```python
from build123d import *

# Parameters (mm, degrees)
F1_R     = 5
F2_R     = 10
F5_DEPTH = 5


with BuildPart() as f3:
    # F1 (on offset) → F3 section 0
    with BuildSketch(Plane.YZ.offset(50)):
        Circle(F1_R)
    # F2 (on Right) → F3 section 1
    with BuildSketch(Plane.YZ):
        Circle(F2_R)
    loft()

    # F4 (on face) → F5 (cut)
    with BuildSketch(Plane.YZ.offset(50)):
        with BuildLine():
            Line((5.64992, 4.784543), (1.451947, 4.784543))
            ThreePointArc((1.451947, 4.784543), (4.016201, 2.978277), (5, 0))
            ThreePointArc((5, 0), (3.684566, -3.379937), (0.430411, -4.98144))
            Line((0.430411, -4.98144), (5.64992, -4.530459))
            Line((5.64992, -4.530459), (5.64992, 3.919373))
            Line((5.64992, 3.919373), (5.64992, 4.784543))
        make_face()
    extrude(amount=-F5_DEPTH, mode=Mode.SUBTRACT)


solid = f3.part
```
Could you check a few things on this model? Use its own coordinates, in mm. Round coordinates to 2 decimals unless told otherwise and drop trailing zeros. Loops run counter-clockwise (first coordinate to the right, second up) from the corner with the lowest first, then second, coordinate; pieces in that order, holes last. Notation, with made-up numbers: M 72,-29 L 97,-29 A24 ccw 97,-16 Z; hole C 67.5,-23 d10. An arc over 180 degrees is marked long. Put each result on its own line as item: value.
Q1. Imagine slicing it at C-C (x = 46). Write out the boundary of the cut face in (y, z).
Check result:
outline: M 0.43,-4.98 A5 ccw 5,0 A5 ccw 1.45,4.78 L 2.5,4.78 A5.4 ccw long 2.46,-4.81 Z
Q2. Imagine slicing it at B-B (x = 6). Write out the boundary of the cut face in (y, z).
Check result:
outline: C 0,0 d18.8
Q3. I need wall thicknesses on probe 1 along X at (y, z) = (4.25, -3); probe 2 along Y at (x, z) = (20, -5.5); probe 3 along Z at (x, y) = (24.5, -6.5). Which ranges of each line are inside material? Lowest first, please.
Check result:
probe 1: 0 to 45
probe 2: -5.81 to 5.81
probe 3: -3.84 to 3.84
Q4. Imagine slicing it at A-A (x = 14). Write out the boundary of the cut face in (y, z).
Check result:
outline: C 0,0 d17.2
Q5. For pin 1 (12 mm diameter, centred on x = 6.5, z = 5, fed in from -Y); pin 2 (1.5 mm diameter, centred on x = 13, y = 1, fed in from -Z); pin 3 (1 mm diameter, centred on x = 28.5, y = -1, fed in from +Z), each with a flat end and sliding along its axis, tell me the tip position at first contact or that it passes through.
Check result:
pin 1: y = -9.75
pin 2: z = -8.74
pin 3: z = 7.16
